Could you check a few things on this drawing? It's one solid part, dimensions in mm from its lowest x, y, z. A direction names the side the tool comes from. Give positions to 0.01 mm unless a question says otherwise; leave off trailing zeros. Write each loop counter-clockwise with the first axis right and the second up, starting at its lowest first coordinate (ties: lowest second). Pieces come first, ordered by that corner, then holes. Notation, with made-up numbers: (20, 44) - (78, 44) arc R15 ccw to (78, 52) - close; hole circle Ø9 at (65.5, 42.25). An arc over 180 degrees is marked (long way). One line per item, written item: value. Start each with the question number.
1) Imagine slicing it at B-B on z = 1.55. Write out the boundary of the cut face in (x, y), plus the area to 3 significant figures.
2) Please list where these lines run through material, in increasing order: L1, parallel to Y at x = 4.5, z = 3.75; L2, parallel to X at y = 4.75, z = 1.3; L3, parallel to Z at x = 2, y = 5.25. Write a range as [from, to].
3) We'd pull the mould along Y, two halves only. Please class the marked faces 5, 6, 7 and 8: +Y half, -Y half, draft (parallel to the pull), parting line (faces both ways), or undercut.
4) On a 3-axis mill with a long thin cutter (end or side, diameter ignored), from which of +Z, -Z, +X, -X, +Y, -Y can I reach the whole of each face in a straight line? I mean the marked faces 1, 2, 3 and 4. Say none if no direction works.
5) Imagine slicing it at A-A on y = 4.5. Write out the boundary of the cut face in (x, z).
6) I'm going to push flat-ended pins straight in: P1, Ø1, axis at y = 3.5, z = 2, coming from the -X side; P2, Ø1.5, axis at x = 3.5, z = 1, coming from the -Y side; P3, Ø0.9, axis at x = 5.5, z = 1.5, coming from the +Y side. Where does each tip first touch, or does it pass through?
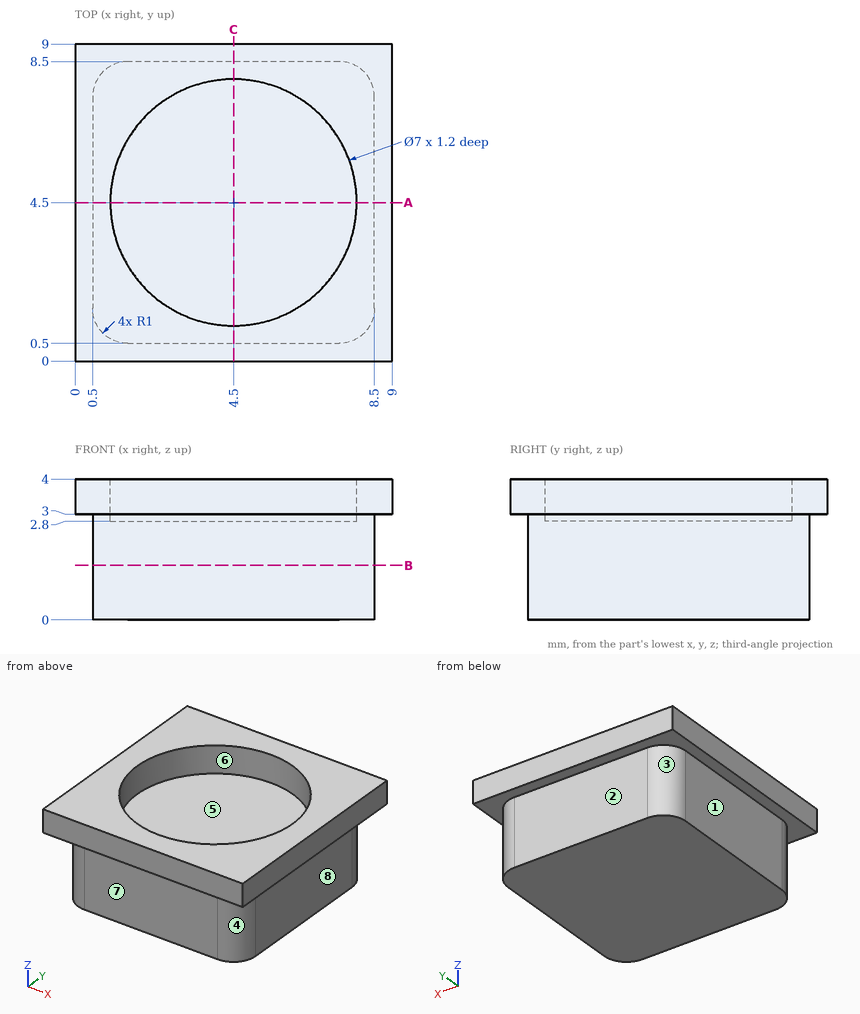
Numbers:
1. outline: (0.5, 1.5) arc R1 ccw to (1.5, 0.5) - (7.5, 0.5) arc R1 ccw to (8.5, 1.5) - (8.5, 7.5) arc R1 ccw to (7.5, 8.5) - (1.5, 8.5) arc R1 ccw to (0.5, 7.5) - close
1. area: 63.1 mm^2
2. L1: [0, 1], [8, 9]
2. L2: [0.5, 8.5]
2. L3: [0, 2.8]
3. face 5: undercut
3. face 6: undercut
3. face 7: -Y half
3. face 8: draft
4. face 1: -Z, -X, +Y, -Y
4. face 2: -Z, +X, -X, +Y
4. face 3: -Z, -X, +Y
4. face 4: -Z, +X, -Y
5. outline: (0, 3) - (0.5, 3) - (0.5, 0) - (8.5, 0) - (8.5, 3) - (9, 3) - (9, 4) - (8, 4) - (8, 2.8) - (1, 2.8) - (1, 4) - (0, 4) - close
6. P1: x = 0.5
6. P2: y = 0.5
6. P3: y = 8.5
